Source: CAD feature listing. Evaluate the final solid. Frame: model axes, mm. Give positions to 0.01 mm unless a question says otherwise; leave off trailing zeros. Loops run counter-clockwise (first coordinate to the right, second up) from the corner with the lowest first, then second, coordinate; pieces in that order, holes last. Notation, with made-up numbers: (-27.5, 33.25) - (-14.5, 33.25) arc R14 ccw to (-14.5, 45.25) - close; hole circle Ø2 at (89.5, 56). An arc over 180 degrees is marked (long way). Put each result on its own line as item: value.
```python
from build123d import *

# Parameters (mm, degrees)
SKETCH_1_R          = 10
EXTRUDE_1_DEPTH     = 2
FILLET_1_R          = 3
SKETCH_2_R          = 1.5
CUT_EXTRUDE_1_DEPTH = 3
SKETCH_3_R          = 1.5
CUT_EXTRUDE_2_DEPTH = 10


with BuildPart() as part:
    # 草图1 → 凸台-拉伸1 (new body)
    with BuildSketch(Plane(origin=(0, 0, 0), x_dir=(1, 0, 0), z_dir=(0, 1, 0))):
        with BuildLine():
            ThreePointArc((-125, -32.5), (-116.213203436, -53.713203436), (-95, -62.5))
            Line((-95, -62.5), (-93, -62.5))
            Line((-93, -62.5), (-93, -27.5))
            Line((-93, -27.5), (-11, -27.5))
            Line((-11, -27.5), (-11, -62.5))
            Line((-11, -62.5), (11, -62.5))
            Line((11, -62.5), (11, -27.5))
            Line((11, -27.5), (93, -27.5))
            Line((93, -27.5), (93, -62.5))
            Line((93, -62.5), (95, -62.5))
            ThreePointArc((95, -62.5), (116.213203436, -53.713203436), (125, -32.5))
            Line((125, -32.5), (125, 32.5))
            ThreePointArc((125, 32.5), (116.213203436, 53.713203436), (95, 62.5))
            Line((95, 62.5), (93, 62.5))
            Line((93, 62.5), (93, 27.5))
            Line((93, 27.5), (11, 27.5))
            Line((11, 27.5), (11, 62.5))
            Line((11, 62.5), (-11, 62.5))
            Line((-11, 62.5), (-11, 27.5))
            Line((-11, 27.5), (-93, 27.5))
            Line((-93, 27.5), (-93, 62.5))
            Line((-93, 62.5), (-95, 62.5))
            ThreePointArc((-95, 62.5), (-116.213203436, 53.713203436), (-125, 32.5))
            Line((-125, 32.5), (-125, -32.5))
        make_face()
        with BuildLine():
            ThreePointArc((-111.5, 30), (-110, 31.5), (-108.5, 30))
            Line((-108.5, 30), (-108.5, -30))
            ThreePointArc((-108.5, -30), (-110, -31.5), (-111.5, -30))
            Line((-111.5, -30), (-111.5, 30))
        make_face(mode=Mode.SUBTRACT)
        with Locations((-80, 0)):
            Circle(SKETCH_1_R, mode=Mode.SUBTRACT)
        with BuildLine():
            ThreePointArc((-69.340891424, -15.009353682), (-70.840891424, -13.509353682), (-69.340891424, -12.009353682))
            Line((-69.340891424, -12.009353682), (-54.340891424, -12.009353682))
            ThreePointArc((-54.340891424, -12.009353682), (-52.840891424, -13.509353682), (-54.340891424, -15.009353682))
            Line((-54.340891424, -15.009353682), (-69.340891424, -15.009353682))
        make_face(mode=Mode.SUBTRACT)
        with BuildLine():
            ThreePointArc((-51.302455724, -1.5), (-52.802455724, 0), (-51.302455724, 1.5))
            Line((-51.302455724, 1.5), (-36.302455724, 1.5))
            ThreePointArc((-36.302455724, 1.5), (-34.802455724, 0), (-36.302455724, -1.5))
            Line((-36.302455724, -1.5), (-51.302455724, -1.5))
        make_face(mode=Mode.SUBTRACT)
        with BuildLine():
            ThreePointArc((-29.892349798, -15.009353682), (-31.392349798, -13.509353682), (-29.892349798, -12.009353682))
            Line((-29.892349798, -12.009353682), (-14.892349798, -12.009353682))
            ThreePointArc((-14.892349798, -12.009353682), (-13.392349798, -13.509353682), (-14.892349798, -15.009353682))
            Line((-14.892349798, -15.009353682), (-29.892349798, -15.009353682))
        make_face(mode=Mode.SUBTRACT)
        with BuildLine():
            ThreePointArc((16.80528281, -15.009353682), (15.30528281, -13.509353682), (16.80528281, -12.009353682))
            Line((16.80528281, -12.009353682), (31.80528281, -12.009353682))
            ThreePointArc((31.80528281, -12.009353682), (33.30528281, -13.509353682), (31.80528281, -15.009353682))
            Line((31.80528281, -15.009353682), (16.80528281, -15.009353682))
        make_face(mode=Mode.SUBTRACT)
        with BuildLine():
            ThreePointArc((53.050737723, -15.009353682), (51.550737723, -13.509353682), (53.050737723, -12.009353682))
            Line((53.050737723, -12.009353682), (68.050737723, -12.009353682))
            ThreePointArc((68.050737723, -12.009353682), (69.550737723, -13.509353682), (68.050737723, -15.009353682))
            Line((68.050737723, -15.009353682), (53.050737723, -15.009353682))
        make_face(mode=Mode.SUBTRACT)
        with BuildLine():
            ThreePointArc((32.314965843, -1.5), (30.814965843, 0), (32.314965843, 1.5))
            Line((32.314965843, 1.5), (47.314965843, 1.5))
            ThreePointArc((47.314965843, 1.5), (48.814965843, 0), (47.314965843, -1.5))
            Line((47.314965843, -1.5), (32.314965843, -1.5))
        make_face(mode=Mode.SUBTRACT)
        with Locations((80, 0)):
            Circle(SKETCH_1_R, mode=Mode.SUBTRACT)
        with BuildLine():
            ThreePointArc((108.5, 30), (110, 31.5), (111.5, 30))
            Line((111.5, 30), (111.5, -30))
            ThreePointArc((111.5, -30), (110, -31.5), (108.5, -30))
            Line((108.5, -30), (108.5, 30))
        make_face(mode=Mode.SUBTRACT)
        with BuildLine():
            ThreePointArc((-69.340891424, 15.971420639), (-70.840891424, 17.471420639), (-69.340891424, 18.971420639))
            Line((-69.340891424, 18.971420639), (-54.340891424, 18.971420639))
            ThreePointArc((-54.340891424, 18.971420639), (-52.840891424, 17.471420639), (-54.340891424, 15.971420639))
            Line((-54.340891424, 15.971420639), (-69.340891424, 15.971420639))
        make_face(mode=Mode.SUBTRACT)
        with BuildLine():
            ThreePointArc((-18.5, 15.971420639), (-20, 17.471420639), (-18.5, 18.971420639))
            Line((-18.5, 18.971420639), (-3.5, 18.971420639))
            ThreePointArc((-3.5, 18.971420639), (-2, 17.471420639), (-3.5, 15.971420639))
            Line((-3.5, 15.971420639), (-18.5, 15.971420639))
        make_face(mode=Mode.SUBTRACT)
        Circle(SKETCH_1_R, mode=Mode.SUBTRACT)
        with BuildLine():
            ThreePointArc((11, 15.821420639), (9.35, 17.471420639), (11, 19.121420639))
            Line((11, 19.121420639), (26, 19.121420639))
            ThreePointArc((26, 19.121420639), (27.65, 17.471420639), (26, 15.821420639))
            Line((26, 15.821420639), (11, 15.821420639))
        make_face(mode=Mode.SUBTRACT)
        with BuildLine():
            ThreePointArc((50.690568566, 15.971420639), (49.190568566, 17.471420639), (50.690568566, 18.971420639))
            Line((50.690568566, 18.971420639), (65.690568566, 18.971420639))
            ThreePointArc((65.690568566, 18.971420639), (67.190568566, 17.471420639), (65.690568566, 15.971420639))
            Line((65.690568566, 15.971420639), (50.690568566, 15.971420639))
        make_face(mode=Mode.SUBTRACT)
    extrude(amount=EXTRUDE_1_DEPTH)

    # 圆角1
    fillet_1_edges = [part.edges().sort_by_distance(p)[0] for p in [
        (-11, 1, -62.5),
        (11, 1, -62.5),
        (11, 1, 62.5),
        (-11, 1, 62.5),
    ]]
    fillet(fillet_1_edges, radius=FILLET_1_R)

    # 草图2 → 切除-拉伸1 (cut, through all)
    with BuildSketch(Plane(origin=(0, 2, 0), x_dir=(1, 0, 0), z_dir=(0, 1, 0))):
        with Locations((107, -55)):
            Circle(SKETCH_2_R)
        with Locations((107, 55)):
            Circle(SKETCH_2_R)
        with Locations((-107, 55)):
            Circle(SKETCH_2_R)
        with Locations((-107, -55)):
            Circle(SKETCH_2_R)
    extrude(amount=-CUT_EXTRUDE_1_DEPTH, mode=Mode.SUBTRACT)

    # 草图3 → 切除-拉伸2 (cut)
    with BuildSketch(Plane.XZ):
        with Locations((0, 55)):
            Circle(SKETCH_3_R)
        with Locations((0, -55)):
            Circle(SKETCH_3_R)
    extrude(amount=-CUT_EXTRUDE_2_DEPTH, mode=Mode.SUBTRACT)


solid = part.part
```
1) Section query C-C, the plane x = -80. Output: boundary loops of the cut face in (y, z), plus the area to 3 significant figures.
Check result:
outline: (0, -27.5) - (2, -27.5) - (2, -10) - (0, -10) - close; (0, 10) - (2, 10) - (2, 27.5) - (0, 27.5) - close
area: 70.0 mm²
2) Material intervals for line 1 along X through (y, z) = (0.4, 25); line 2 along Z through (x, y) = (-15.5, 0.5); line 3 along X through (y, z) = (0.85, 28.5), sorted ascending. Write a range as [from, to].
Check result:
line 1: [-125, -111.5], [-108.5, 108.5], [111.5, 125]
line 2: [-27.5, -18.97], [-15.97, 12.01], [15.01, 27.5]
line 3: [-125, -111.5], [-108.5, -93], [-11, 11], [93, 108.5], [111.5, 125]
3) Mould query, pull axis Z, two halves, no side actions, for faces 1 (the cylindrical face through (115.979, 0.986, 53.945)), 2 (the cylindrical face through (116.445, 0.986, -53.479)), 3 (the cylindrical face through (70, 1, 0)). Classes: pulls with the +Z half, pulls with the -Z half, needs draft (parallel to the pull), parting line crosses it, or undercut.
Check result:
face 1: pulls with the +Z half
face 2: pulls with the -Z half
face 3: undercut
4) Section query B-B, the plane z = -50. Output: boundary loops of the cut face in (x, y), plus the area to 3 significant figures.
Check result:
outline: (-119.37, 0) - (-93, 0) - (-93, 2) - (-119.37, 2) - close; (-11, 0) - (11, 0) - (11, 2) - (-11, 2) - close; (93, 0) - (119.37, 0) - (119.37, 2) - (93, 2) - close
area: 149 mm²
5) Section query D-D, the plane z = 4. Output: boundary loops of the cut face in (x, y).
Check result:
outline: (-125, 0) - (-111.5, 0) - (-111.5, 2) - (-125, 2) - close; (-108.5, 0) - (-89.17, 0) - (-89.17, 2) - (-108.5, 2) - close; (-70.83, 0) - (-9.17, 0) - (-9.17, 2) - (-70.83, 2) - close; (9.17, 0) - (70.83, 0) - (70.83, 2) - (9.17, 2) - close; (89.17, 0) - (108.5, 0) - (108.5, 2) - (89.17, 2) - close; (111.5, 0) - (125, 0) - (125, 2) - (111.5, 2) - close
6) Pin query (flat end, axial travel): P1, Ø18, axis at x = -80, z = 0, coming from the +Y side; P2, Ø1, axis at y = 0.5, z = 51.5, coming from the +X side; P3, Ø1, axis at x = 15, y = 1, coming from the +Z side; P4, Ø0.6, axis at y = 0.5, z = -43.5, coming from the +X side. Return the tip coordinate at first contact, or that it passes through.
Check result:
P1: through
P2: x = 118.62
P3: z = 27.5
P4: x = 123.03
7) Section query A-A, the plane x = 58. Output: boundary loops of the cut face in (y, z), plus the area to 3 significant figures.
Check result:
outline: (0, -27.5) - (2, -27.5) - (2, -18.97) - (0, -18.97) - close; (0, -15.97) - (2, -15.97) - (2, 12.01) - (0, 12.01) - close; (0, 15.01) - (2, 15.01) - (2, 27.5) - (0, 27.5) - close
area: 98.0 mm²
